```python
from build123d import *

# Parameters (mm, degrees)
SKETCH1_R               = 2
FORMA_B_SICA_DEPTH      = 5
FORMA_B_SICA_2_DEPTH    = 5
BOSS_EXTRUDE2_DEPTH     = 23.3
CARRIL_CREMALLERA_DEPTH = 56.7
ELIMINAR_FILETE_DEPTH   = 23.3
FILLET2_R               = 2


with BuildPart() as part:
    # Sketch1 → Forma básica (new body)
    with BuildSketch(Plane.XY):
        with BuildLine():
            ThreePointArc((-25.85, -9.9), (-27.617766953, -9.167766953), (-28.35, -7.4))
            Line((-28.35, -7.4), (-28.35, 9.9))
            Line((-28.35, 9.9), (-20.15, 9.9))
            Line((-20.15, 9.9), (-20.15, -9.9))
            Line((-20.15, -9.9), (-25.85, -9.9))
        make_face()
        with Locations((-24.25, -5)):
            Circle(SKETCH1_R, mode=Mode.SUBTRACT)
        with Locations((-24.25, 5)):
            Circle(SKETCH1_R, mode=Mode.SUBTRACT)
    extrude(amount=FORMA_B_SICA_DEPTH)



with BuildPart() as body_2:
    # Sketch1 → Forma b_sica 2 (new body)
    with BuildSketch(Plane.XY):
        with BuildLine():
            ThreePointArc((28.35, -7.4), (27.617766953, -9.167766953), (25.85, -9.9))
            Line((25.85, -9.9), (20.15, -9.9))
            Line((20.15, -9.9), (20.15, 9.9))
            Line((20.15, 9.9), (28.35, 9.9))
            Line((28.35, 9.9), (28.35, -7.4))
        make_face()
        with Locations((24.25, 5)):
            Circle(SKETCH1_R, mode=Mode.SUBTRACT)
        with Locations((24.25, -5)):
            Circle(SKETCH1_R, mode=Mode.SUBTRACT)
    extrude(amount=FORMA_B_SICA_2_DEPTH)


with BuildPart() as part_1:
    add(part.part)

    add(body_2.part)  # Boss-Extrude2 merges body 2
    # Sketch1<3> → Boss-Extrude2 (add)
    with BuildSketch(Plane.XY):
        with BuildLine():
            Line((-28.35, 9.9), (-20.15, 9.9))
            Line((-20.15, 9.9), (20.15, 9.9))
            Line((20.15, 9.9), (28.35, 9.9))
            Line((28.35, 9.9), (28.35, 17.4))
            ThreePointArc((28.35, 17.4), (27.617766953, 19.167766953), (25.85, 19.9))
            Line((25.85, 19.9), (-25.85, 19.9))
            ThreePointArc((-25.85, 19.9), (-27.617766953, 19.167766953), (-28.35, 17.4))
            Line((-28.35, 17.4), (-28.35, 9.9))
        make_face()
    extrude(amount=BOSS_EXTRUDE2_DEPTH)

    # Sketch2 → Carril cremallera (add)
    with BuildSketch(Plane(origin=(28.35, 0, 0), x_dir=(0, 0, -1), z_dir=(1, 0, 0))):
        Polygon((-23.3, 19.9), (-19.623044738, 23.576955262), (-19.623044738, 28.776955262), (-36.123044738, 28.776955262), (-36.123044738, 23.576955262), (-32.446089476, 19.9), (-40.446089476, 19.9), (-40.446089476, 33.9), (-15.3, 33.9), (-15.3, 19.9), align=None)
    extrude(amount=-CARRIL_CREMALLERA_DEPTH)

    # Sketch3 → Eliminar filete (add)
    with BuildSketch(Plane.XY.offset(23.3)):
        with BuildLine():
            Line((-28.35, 17.4), (-28.35, 19.9))
            Line((-28.35, 19.9), (-25.85, 19.9))
            ThreePointArc((-25.85, 19.9), (-27.617766953, 19.167766953), (-28.35, 17.4))
        make_face()
        with BuildLine():
            Line((28.35, 19.9), (25.85, 19.9))
            ThreePointArc((25.85, 19.9), (27.617766953, 19.167766953), (28.35, 17.4))
            Line((28.35, 17.4), (28.35, 19.9))
        make_face()
    extrude(amount=-ELIMINAR_FILETE_DEPTH)

    # Fillet2
    fillet2_edges = [part_1.edges().sort_by_distance(p)[0] for p in [
        (28.35, 33.9, 27.873044738),
        (-28.35, 33.9, 27.873044738),
        (-28.35, 19.9, 7.65),
        (28.35, 19.9, 7.65),
    ]]
    fillet(fillet2_edges, radius=FILLET2_R)


solid = part_1.part
```
Read the model definition and answer for the solid it produces. Units are mm, in the model's axes. A direction names the side the tool comes from. Give positions to 0.01 mm unless a question says otherwise; leave off trailing zeros. Write each loop counter-clockwise with the first axis right and the second up, starting at its lowest first coordinate (ties: lowest second). Pieces come first, ordered by that corner, then holes. Notation, with made-up numbers: (47, 65) -> (87, 65) arc R14 ccw to (87, 82) -> close; hole circle Ø11 at (-36, -30.5). An arc over 180 degrees is marked (long way). Answer in a Markdown table with one row per item.
1) A tool of negligible diameter and unlimited length cuts with its end or side. For faces 1 (the flat face through (-20.15, 0, 2)), 2 (the flat face through (0, 26, 36.123)), 3 (the flat face through (0, 9.9, 11)), 4 (the flat face through (24, 0, 5)), 5 (the flat face through (0, 19.9, 8)), from which of +Z, -Z, +X, -X, +Y, -Y can it reach the whole face along a straight path? Write none if from no direction.
Results list:
| item | result |
|---|---|
| face 1 | +Z, -Z, -Y |
| face 2 | +X, -X |
| face 3 | +Z, -Y |
| face 4 | +Z, +X, -X, -Y |
| face 5 | -Z, +X, -X, +Y |
2) Section C-C on y = 5 is taken. Give the vertices of the cut face in (x, z), plus the area to 3 significant figures.
Results list:
| item | result |
|---|---|
| outline | (-28.35, 0) -> (-26.25, 0) -> (-26.25, 5) -> (-28.35, 5) -> close; (-22.25, 0) -> (-20.15, 0) -> (-20.15, 5) -> (-22.25, 5) -> close; (20.15, 0) -> (22.25, 0) -> (22.25, 5) -> (20.15, 5) -> close; (26.25, 0) -> (28.35, 0) -> (28.35, 5) -> (26.25, 5) -> close |
| area | 42.0 mm^2 |
3) Each of these flat-tipped pins is pushed along its axis until it touches: pin 1 Ø5 at (y, z) = (21, 5) entering from +X; pin 2 Ø5 at (x, z) = (-14, 30.5) entering from -Y; pin 3 Ø12 at (x, z) = (14.5, 9.5) entering from -Y. Where does it stop, or does it pass through?
Results list:
| item | result |
|---|---|
| pin 1 | x = 28.26 |
| pin 2 | y = 19.9 |
| pin 3 | y = 9.9 |
4) Straight lines are drawn through the part: line 1 (Y direction, x = -24.25, z = 3.3); line 2 (Z direction, x = 7, y = 26); line 3 (Z direction, x = 25.5, y = 16). For each, find the intervals that lie inside material, in ascending order. Write a range as [from, to].
Results list:
| item | result |
|---|---|
| line 1 | [-9.9, -7], [-3, 3], [7, 19.9] |
| line 2 | [15.3, 19.62], [36.12, 40.45] |
| line 3 | [0, 23.3] |
5) Section B-B on y = 0.5 is taken. Give the vertices of the cut face in (x, z), plus the area to 3 significant figures.
Results list:
| item | result |
|---|---|
| outline | (-28.35, 0) -> (-20.15, 0) -> (-20.15, 5) -> (-28.35, 5) -> close; (20.15, 0) -> (28.35, 0) -> (28.35, 5) -> (20.15, 5) -> close |
| area | 82.0 mm^2 |
6) Section A-A on x = -24.25 is taken. Give the vertices of the cut face in (y, z), plus the area to 3 significant figures.
Results list:
| item | result |
|---|---|
| outline | (-9.9, 0) -> (-7, 0) -> (-7, 5) -> (-9.9, 5) -> close; (-3, 0) -> (3, 0) -> (3, 5) -> (-3, 5) -> close; (7, 0) -> (19.9, 0) -> (19.9, 15.3) -> (33.9, 15.3) -> (33.9, 40.45) -> (19.9, 40.45) -> (19.9, 32.45) -> (23.58, 36.12) -> (28.78, 36.12) -> (28.78, 19.62) -> (23.58, 19.62) -> (19.9, 23.3) -> (9.9, 23.3) -> (9.9, 5) -> (7, 5) -> close |
| area | 511 mm^2 |
7) Section D-D on z = 25.5 is taken. Give the vertices of the cut face in (x, y).
Results list:
| item | result |
|---|---|
| outline | (-28.35, 28.78) -> (28.35, 28.78) -> (28.35, 31.9) arc R2 ccw to (26.35, 33.9) -> (-26.35, 33.9) arc R2 ccw to (-28.35, 31.9) -> close |
8) Determine the mould class of faces 6 (the flat face through (-23, -9.9, 2)), 7 (the cylindrical face through (-27.78, 19.3, 7.54)), 8 (the cylindrical face through (-26.248, 5.088, 2.465)) for opening direction X: released by +X, released by -X, zero draft, split by the parting line, or undercut.
Results list:
| item | result |
|---|---|
| face 6 | zero draft |
| face 7 | released by -X |
| face 8 | undercut |
